Autodesk Inventor part; units mm, degrees
ref_plane "Work Plane1" through (0, -6.5, 0) normal (0, 1, 0) x (-1, 0, 0)
ref_plane "Work Plane2" through (-4.375, -6.5, 6.125) normal (0, 0, -1) x (-1, 0, 0)
ref_plane "YZ Plane" through (0, 0, 0) normal (1, 0, 0) x (0, 1, 0)
ref_plane "Work Plane1" through (0, -6.5, 0) normal (0, 1, 0) x (-1, 0, 0)
sketch "Sketch1" plane through (0, -6.5, 0) normal (0, 1, 0) x (-1, 0, 0)
  arc A0 (-2.625, 0) -> (0, -2.625) centre (0, 0) ccw
  line L0 (-2.625, 0) -> (-2.625, 26.85)
  arc A1 (0, 29.475) -> (-2.625, 26.85) centre (0, 26.85) ccw
  line L1 (4.375, 26.85) -> (4.375, 14.875)
  line L2 (16.75, 9.625) -> (4.375, 9.625)
  line L3 (0, 29.475) -> (1.75, 29.475)
  line L4 (4.375, 9.625) -> (4.375, 2.625)
  arc A2 (4.375, 26.85) -> (1.75, 29.475) centre (1.75, 26.85) ccw
  line L5 (4.375, 14.875) -> (16.75, 14.875)
  line L6 (16.75, -2.625) -> (0, -2.625)
  arc A3 (16.75, 9.625) -> (16.75, 14.875) centre (16.75, 12.25) ccw
  line L7 (4.375, 2.625) -> (16.75, 2.625)
  arc A4 (16.75, -2.625) -> (16.75, 2.625) centre (16.75, 0) ccw
  dimension "d35" = 7
  dimension "d36" = 7
  dimension "d37" = 12.375
  dimension "d38" = 5.25
  dimension "d39" = 14.6
extrude "Extrusion2" add sketch "Sketch1" along normal blind 13
hole "Hole3" at (-12.875, 0, 9.625) direction (0, 0, 1) diameter 2.529 depth 5.25
sketch "Sketch3" plane through (-4.375, -6.5, 9.625) normal (0, 0, -1) x (-1, 0, 0)
  point P0 (8.5, 6.5)
hole "Hole1" at (-12.875, 0, -2.625) direction (0, 0, 1) diameter 2.529 depth 5.25
sketch "Sketch6" plane through (-16.75, -6.5, 14.875) normal (0, 0, 1) x (1, 0, 0)
  circle A0 centre (-4.0623, 15.5) radius 4.5
  circle A1 centre (3.875, 6.5) radius 4.5
  circle A2 centre (3.875, 6.5) radius 1.2645
  line L0 (0, 0) -> (12.375, 0)
  line L1 (12.375, 0) -> (12.375, 13)
  line L2 (0, 13) -> (12.375, 13)
  line L3 (0, 0) -> (0, 13)
  circle A3 centre (3.875, 6.5) radius 1.2645
  circle A4 centre (-4.0623, 15.5) radius 6.5
  circle A5 centre (3.875, 6.5) radius 6.5
  line L4 (3.875, 11) -> (-4.0623, 11)
  line L5 (0, 0) -> (0, 0)
  line L6 (0, 0) -> (0, 13)
  line L7 (0, 13) -> (0, 13)
  line L8 (0, 0) -> (0, 13)
  line L9 (-2.625, 0) -> (-2.625, 13)
  line L10 (-2.625, 0) -> (-15.6685, 13.1351)
  line L11 (-15.6685, 13.1351) -> (-1.6162, 27.0894)
  line L12 (12.375, 0) -> (12.375, 13)
  line L13 (-1.6162, 27.0894) -> (12.375, 13)
  line L14 (2.9639, 22.4772) -> (-11.0884, 8.5228)
  circle A6 centre (-4.0623, 15.5) radius 1.2645
  point P0 (16.75, 6.5)
  point P1 (-2.625, 11)
  point P2 (-0.8154, 11)
  point P3 (0, 11.7187)
  dimension "d26" = 9
  dimension "d27" = 9
  dimension "d28" = 2
  dimension "d29" = 2
  dimension "d30" = 1
extrude "Extrusion4" add sketch "Sketch6" against normal up to surface (5.25 mm away) contours A0 L14 A6 | A0 L14 A4 L2 L3 A5 L4 L9 | L14 A6 A0 | A0 L14 A4 | L9 L4 A0 | A0 L4 L9 A4 L14 | L14 L13 L2 A4 | A4 L11 L13 L14 | L14 L10 L11 A4 | A4 L9 L10 L14
sketch "Sketch7" plane through (0, -6.5, 0) normal (0, -1, 0) x (1, 0, 0)
  arc A0 (0, -2.625) -> (2.625, 0) centre (0, 0) ccw
  line L0 (2.625, 26.85) -> (2.625, 0)
  arc A1 (2.625, 26.85) -> (0, 29.475) centre (0, 26.85) ccw
  line L1 (-1.75, 29.475) -> (0, 29.475)
  arc A2 (-1.75, 29.475) -> (-4.375, 26.85) centre (-1.75, 26.85) ccw
  line L2 (-4.375, 14.875) -> (-4.375, 26.85)
  line L3 (-16.75, 14.875) -> (-4.375, 14.875)
  arc A3 (-16.75, 14.875) -> (-19.375, 12.25) centre (-16.75, 12.25) ccw
  arc A4 (-19.375, 12.25) -> (-16.75, 9.625) centre (-16.75, 12.25) ccw
  line L4 (-4.375, 9.625) -> (-16.75, 9.625)
  line L5 (-4.375, 2.625) -> (-4.375, 9.625)
  line L6 (-16.75, 2.625) -> (-4.375, 2.625)
  arc A5 (-16.75, 2.625) -> (-16.75, -2.625) centre (-16.75, 0) ccw
  line L7 (0, -2.625) -> (-16.75, -2.625)
  arc A6 (-17.5654, 14.7451) -> (-19.375, 12.25) centre (-16.75, 12.25) ccw
  line L8 (-17.5654, 14.875) -> (-17.5654, 14.7451)
  line L9 (-19.375, 14.875) -> (-17.5654, 14.875)
  line L10 (-19.375, 14.875) -> (-19.375, 12.25)
  line L11 (-32.4185, 9.625) -> (-19.375, 9.625)
  line L12 (-19.375, 12.25) -> (-19.375, 9.625)
  line L13 (-19.375, 14.875) -> (-19.375, 12.25)
  line L14 (-32.4185, 14.875) -> (-19.375, 14.875)
  line L15 (-32.4185, 14.875) -> (-32.4185, 9.625)
  arc A7 (-19.375, 12.25) -> (-17.5654, 9.7549) centre (-16.75, 12.25) ccw
  line L16 (-19.375, 12.25) -> (-19.375, 9.625)
  line L17 (-19.375, 9.625) -> (-17.5654, 9.625)
  line L18 (-17.5654, 9.7549) -> (-17.5654, 9.625)
  line L19 (-17.5654, 9.7549) -> (-17.5654, 9.625)
  line L20 (-17.5654, 9.625) -> (-16.75, 9.625)
  line L21 (-17.5654, 14.875) -> (-16.75, 14.875)
  line L22 (-17.5654, 14.875) -> (-17.5654, 14.7451)
  point P0 (-16.75, 9.625)
extrude "Extrusion5" add sketch "Sketch7" against normal blind 15 contours L20 L18 A4 | L18 L17 L12 A4 | A3 L8 L21 | L10 L9 L8 A3
ref_plane "Work Plane2" through (-4.375, -6.5, 6.125) normal (0, 0, -1) x (-1, 0, 0)
mirror "Mirror1" about plane through (-4.375, -6.5, 6.125) normal (0, 0, -1) of "Extrusion4", "Extrusion5"
fillet "Fillet1" radius 8.35 4 edges at (-32.4185, 6.6351, 12.25) (-18.3662, 20.5894, 12.25) (-18.3662, 20.5894, 0) (-32.4185, 6.6351, 0)
sketch "Sketch8" plane through (-4.375, -6.5, 2.625) normal (-1, 0, 0) x (0, 0, 1)
  line L0 (0, 0) -> (7, 0)
  line L1 (7, 0) -> (7, 13)
  line L2 (0, 13) -> (7, 13)
  line L3 (0, 0) -> (0, 13)
  line L4 (0, 0) -> (0, 13)
  line L5 (0, 6.5) -> (7, 6.5)
  line L6 (7, 0) -> (7, 13)
  point P0 (-2.625, 6.5)
  point P1 (3.5, 6.5)
hole "Hole5" at (-4.375, 0, 6.125) direction (1, 0, 0) diameter 3.6 end through all counterbore diameter 6.5 counterbore depth 3
sketch "Sketch5" plane through (0, -6.5, -2.625) normal (0, 0, -1) x (-1, 0, 0)
  point P0 (12.875, 6.5)
properties part number "Idle belt holder"
Part model, mm, in its own coordinate system. A direction names the side the tool comes from. Round coordinates to 2 decimals unless told otherwise and drop trailing zeros. Loops run counter-clockwise (first coordinate to the right, second up) from the corner with the lowest first, then second, coordinate; pieces in that order, holes last. Notation, with made-up numbers: (-24, 61) -> (6, 61) arc R31 cw to (6, 95) -> close; hole circle Ø2 at (71, 22). An arc over 180 degrees is marked (long way). Use one line per item in the form item = value. Start each with the question number.
Item 1: Drill centre lines: line 1 along Z through (x, y) = (-22.5, 14) (3 decimals); line 2 along Z through (x, y) = (-0.5, 0) (3 decimals); line 3 along X through (y, z) = (1.75, 7.5) (3 decimals). Where is each one in solid material? Low to high.
Item 2: Band-saw the part on A-A (y = 0). Give the number of separate pieces and of enclosed holes in the cut face, plus the area to 3 significant figures.
Item 3: Band-saw the part on B-B (x = -17). List the corners of the cut face in (y, z) (3 decimals), plus the area to 3 significant figures.
Item 4: Two-plate mould, pull along Y, no slides. Class faces 5 (the flat face through (-15, 5, -2.625)), 6 (the cylindrical face through (-21.086, 7.766, 12.287)), 7 (the flat face through (-1.375, 1, 8)), 8 (the cylindrical face through (-18.29, 17.13, 0.04)): released by +Y, released by -Y, zero draft, split by the parting line, or undercut.
Item 5: Tool access for faces 1 (the cylindrical face through (-2.854, -0.976, 9.225)), 2 (the flat face through (-4.375, 0, 21)), 3 (the flat face through (-17, 5, 9.625)), 4 (the flat face through (-1, 6.5, 14)): list every direction of +Z, -Z, +X, -X, +Y, -Y with a clear straight run to the whole face (end or side of a thin tool).
Item 6: Drop flat-ended pins along their axis: pin 1 Ø6 at (y, z) = (14.5, 8) entering from +X; pin 2 Ø10 at (y, z) = (5.5, 9.5) entering from -X; pin 3 Ø2 at (x, z) = (1, 21) entering from +Y; pin 4 Ø7 at (y, z) = (1.5, 5.5) entering from -X. Give the stop position or say it passes through.
Item 7: Band-saw the part on D-D (z = 26). List the corners of the cut face in (x, y) (3 decimals).
Data:
q1.line_1 = -2.625 to 2.625, 9.625 to 14.875
q1.line_2 = -2.625 to 4.325, 7.925 to 29.475
q1.line_3 = -1.375 to 2.625
q2.separate_pieces = 4
q2.enclosed_holes = 0
q2.area = 385 mm^2
q3.outline = (-6.5, -2.625) -> (17.011, -2.625) -> (17.011, 2.625) -> (-6.5, 2.625) -> close; (-6.5, 9.625) -> (17.011, 9.625) -> (17.011, 14.875) -> (-6.5, 14.875) -> close
q3.area = 247 mm^2
q4.face_5 = zero draft
q4.face_6 = undercut
q4.face_7 = undercut
q4.face_8 = released by +Y
q5.face_1 = -X
q5.face_2 = +Z, -X, +Y, -Y
q5.face_3 = -X, +Y, -Y
q5.face_4 = +Z, -Z, +X, +Y
q6.pin_1 = -9.82
q6.pin_2 = -28.96
q6.pin_3 = 6.5
q6.pin_4 = -28.36
q7.outline = (-4.375, -6.5) -> (2.625, -6.5) -> (2.625, 6.5) -> (-4.375, 6.5) -> close
